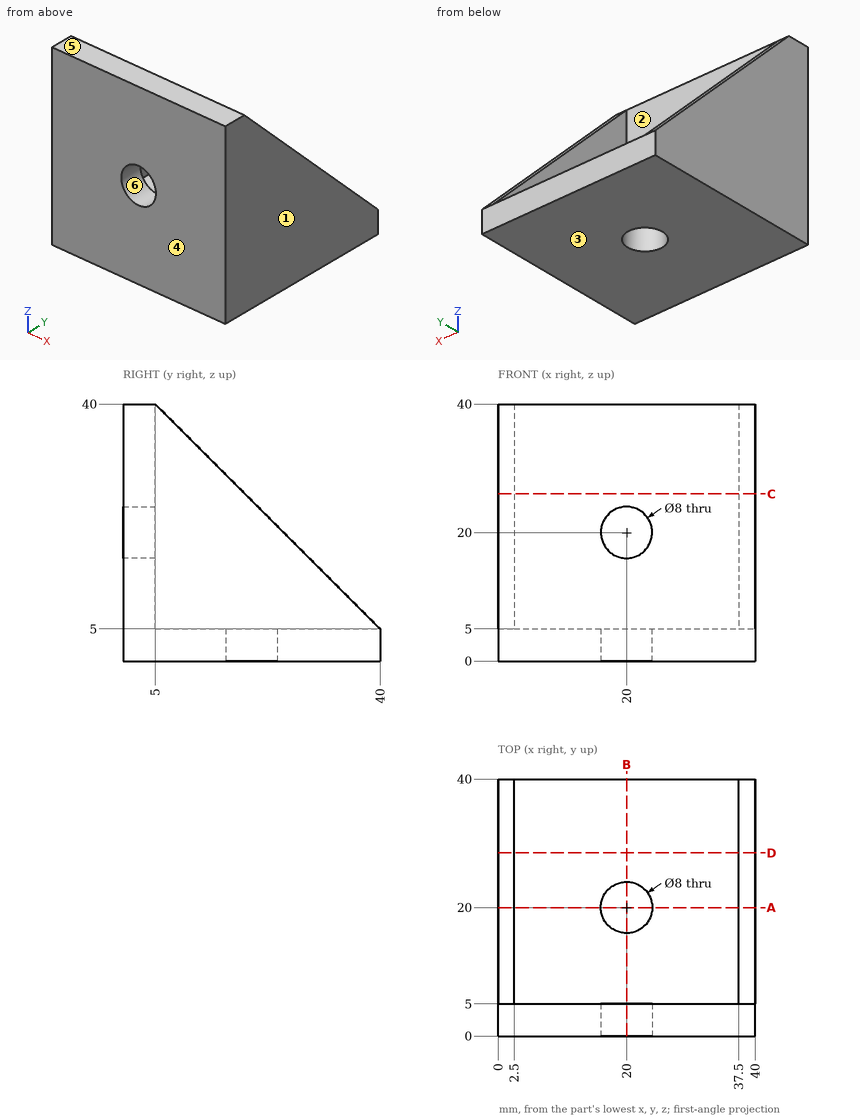
Job drawing, mm, ordinate dimensions from the low corner. One solid piece. A direction names the side the tool comes from. Round coordinates to 2 decimals unless told otherwise and drop trailing zeros. Write each loop counter-clockwise with the first axis right and the second up, starting at its lowest first coordinate (ties: lowest second). Pieces come first, ordered by that corner, then holes. Notation, with made-up numbers: M 86,79 L 135,79 A16 ccw 135,103 Z; hole C -25,-25.75 d3. An arc over 180 degrees is marked long. Return JSON: item names as keys, results as strings. Group by question number.
(1) Two-plate mould, pull along Z, no slides. Class the marked faces 3, 4, 5 and 6: +Z half, -Z half, draft (parallel to the pull), parting line (faces both ways), or undercut.
(2) Which spindle directions (+Z, -Z, +X, -X, +Y, -Y) get a long thin tool onto all of the face, cutting with end or side? Do the marked faces 1 and 2. Say none if no direction does.
(3) Saw through at C-C on z = 26. Write the cut outline in (x, y), then the cut area to 3 significant figures.
(4) Pin check, flat tips, straight feed: pin 1 Ø1.5 at (x, y) = (19, 22.5) entering from +Z; pin 2 Ø17.5 at (x, z) = (27.5, 16) entering from +Y; pin 3 Ø4 at (x, y) = (26, 10) entering from +Z. Stop position of each tip, or through.
(5) Saw through at D-D on y = 28.5. Write the cut outline in (x, z), then the cut area to 4 significant figures.
(6) Saw through at A-A on y = 20. Write the cut outline in (x, z).
(7) Saw through at B-B on x = 20. Write the cut outline in (y, z), then the cut area to 3 significant figures.
(8) Drill centre line: probe 1 along X at (y, z) = (20, 1). Where is it in solid material? Low to high.
Returned:
{
 "1": {"face 3": "-Z half", "face 4": "draft", "face 5": "+Z half", "face 6": "undercut"},
 "2": {"face 1": "+Z, -Z, +X, +Y, -Y", "face 2": "+Z, +Y"},
 "3": {"outline": "M 0,0 L 40,0 L 40,19 L 37.5,19 L 37.5,5 L 2.5,5 L 2.5,19 L 0,19 Z", "area": "270 mm²"},
 "4": {"pin 1": "through", "pin 2": "y = 5", "pin 3": "z = 5"},
 "5": {"outline": "M 0,0 L 40,0 L 40,16.5 L 37.5,16.5 L 37.5,5 L 2.5,5 L 2.5,16.5 L 0,16.5 Z", "area": "257.5 mm²"},
 "6": {"outline": "M 0,0 L 16,0 L 16,5 L 2.5,5 L 2.5,25 L 0,25 Z; M 24,0 L 40,0 L 40,25 L 37.5,25 L 37.5,5 L 24,5 Z"},
 "7": {"outline": "M 0,0 L 16,0 L 16,5 L 5,5 L 5,16 L 0,16 Z; M 0,24 L 5,24 L 5,40 L 0,40 Z; M 24,0 L 40,0 L 40,5 L 24,5 Z", "area": "295 mm²"},
 "8": {"probe 1": "0 to 16, 24 to 40"}
}
